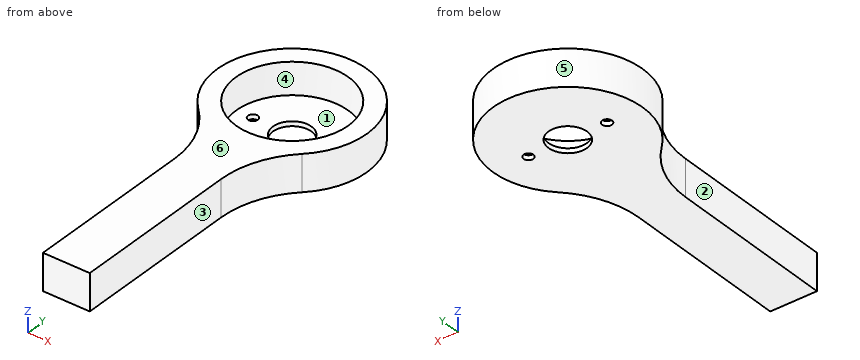
from build123d import *

# Parameters (mm, degrees)
SKETCH1_R           = 6
BOSS_EXTRUDE1_DEPTH = 3.9
SKETCH5_R           = 8
SKETCH5_R_2         = 2.05
SKETCH5_R_3         = 0.525
BOSS_EXTRUDE3_DEPTH = 0.5


with BuildPart() as part:
    # Sketch1 → Boss-Extrude1 (new body)
    with BuildSketch(Plane.XY):
        with BuildLine():
            Line((-2.5, -31), (2.5, -31))
            Line((2.5, -31), (2.5, -12.951833847))
            ThreePointArc((2.5, -12.951833847), (3.295532486, -9.043154047), (5.555555556, -5.756370599))
            ThreePointArc((5.555555556, -5.756370599), (0, 8), (-5.555555556, -5.756370599))
            ThreePointArc((-5.555555556, -5.756370599), (-3.295532486, -9.043154047), (-2.5, -12.951833847))
            Line((-2.5, -12.951833847), (-2.5, -31))
        make_face()
        Circle(SKETCH1_R, mode=Mode.SUBTRACT)
    extrude(amount=BOSS_EXTRUDE1_DEPTH)

    # Sketch5 → Boss-Extrude3 (add)
    with BuildSketch(Plane(origin=(0, 0, 0), x_dir=(-1, 0, 0), z_dir=(0, 0, -1))):
        Circle(SKETCH5_R)
        Circle(SKETCH5_R_2, mode=Mode.SUBTRACT)
        with Locations((4.2, 0)):
            Circle(SKETCH5_R_3, mode=Mode.SUBTRACT)
        with Locations((-4.2, 0)):
            Circle(SKETCH5_R_3, mode=Mode.SUBTRACT)
    extrude(amount=-BOSS_EXTRUDE3_DEPTH)


solid = part.part
Input: part model. Units: mm. Frame: model coordinates. Face numbers are marked on the shaded views. A direction names the side the tool comes from. Coordinates: 2 decimals unless noted, no trailing zeros. Order: outer loops, then holes, each group sorted by start corner. A loop starts at its lowest first (then second) coordinate and runs counter-clockwise, first axis right, second up. Notation, with made-up numbers: M 3.25,-12.5 L 31.25,-12.5 A29 cw 31.25,9.5 Z; hole C 43.5,9 d9. An arc over 180 degrees is marked long. Answer in a Markdown table with one row per item.
(1) Draft query along X for the marked faces 4, 5 and 6. Return one class per face: pulls with the +X half, pulls with the -X half, needs draft (parallel to the pull), parting line crosses it, or undercut.
Numbers:
| item | result |
|---|---|
| face 4 | undercut |
| face 5 | parting line crosses it |
| face 6 | needs draft |
(2) Section query D-D, the plane y = 5.5. Output: boundary loops of the cut face in (x, z).
Numbers:
| item | result |
|---|---|
| outline | M -5.81,0 L 5.81,0 L 5.81,3.9 L 2.4,3.9 L 2.4,0.5 L -2.4,0.5 L -2.4,3.9 L -5.81,3.9 Z |
(3) Access query for the marked faces 1, 2 and 3. Directions: +Z, -Z, +X, -X, +Y, -Y. A direction counts if a zero-diameter tool reaches every point of the face in a straight line with its end or side. Return the directions, or none.
Numbers:
| item | result |
|---|---|
| face 1 | +Z |
| face 2 | +Z, -Z, -X, -Y |
| face 3 | +Z, -Z, +X, -Y |
(4) Section query C-C, the plane y = 0. Output: boundary loops of the cut face in (x, z) (3 decimals).
Numbers:
| item | result |
|---|---|
| outline | M -8,0 L -4.725,0 L -4.725,0.5 L -6,0.5 L -6,3.9 L -8,3.9 Z; M -3.675,0 L -2.05,0 L -2.05,0.5 L -3.675,0.5 Z; M 2.05,0 L 3.675,0 L 3.675,0.5 L 2.05,0.5 Z; M 4.725,0 L 8,0 L 8,3.9 L 6,3.9 L 6,0.5 L 4.725,0.5 Z |
(5) Section query B-B, the plane x = 0. Output: boundary loops of the cut face in (y, z), plus the area to 3 significant figures.
Numbers:
| item | result |
|---|---|
| outline | M -31,0 L -2.05,0 L -2.05,0.5 L -6,0.5 L -6,3.9 L -31,3.9 Z; M 2.05,0 L 8,0 L 8,3.9 L 6,3.9 L 6,0.5 L 2.05,0.5 Z |
| area | 109 mm^2 |
(6) Section query A-A, the plane z = 0.9. Output: boundary loops of the cut face in (x, y), plus the area to 3 significant figures.
Numbers:
| item | result |
|---|---|
| outline | M -5.56,-5.76 A10 cw -2.5,-12.95 L -2.5,-31 L 2.5,-31 L 2.5,-12.95 A10 cw 5.56,-5.76 A8 ccw long Z; hole C 0,0 d12 |
| area | 211 mm^2 |
(7) Contact query for flat-ended pins moving along their axis: pin 1 Ø2 at (y, z) = (-23.5, 1) entering from -X; pin 2 Ø2 at (y, z) = (-22, 2.5) entering from +X; pin 3 Ø1 at (x, z) = (-5.5, 1.5) entering from +Y (3 decimals). Output: stop coordinate, or through.
Numbers:
| item | result |
|---|---|
| pin 1 | stops at x = -2.5 |
| pin 2 | stops at x = 2.5 |
| pin 3 | stops at y = 6.245 |
(8) Material intervals for line 1 (Y direction, x = 0, z = 1.3); line 2 (X direction, y = 0, z = 3.25); line 3 (Z direction, x = 1.5, y = -2), sorted ascending. Write a range as [from, to].
Numbers:
| item | result |
|---|---|
| line 1 | y = [-31, -6], [6, 8] |
| line 2 | x = [-8, -6], [6, 8] |
| line 3 | z = [0, 0.5] |
